Autodesk Inventor part; units mm, degrees
ref_plane "YZ Plane" through (0, 0, 0) normal (1, 0, 0) x (0, 1, 0)
ref_plane "XZ Plane" through (0, 0, 0) normal (0, 1, 0) x (-1, 0, 0)
ref_plane "XY Plane" through (0, 0, 0) normal (0, 0, 1) x (1, 0, 0)
sketch "Sketch1" plane through (0, 0, 0) normal (0, 0, 1) x (1, 0, 0)
  circle A0 centre (0, 0) radius 1.5
  circle A1 centre (-42, 0) radius 1.5
  circle A2 centre (0, -36) radius 1.5
  arc A3 (-42, 7.5) -> (-42, -7.5) centre (-42, 0) ccw
  line L0 (-42, 1.5) -> (-42, -1.5)
  arc A4 (-6, -36) -> (6, -36) centre (0, -36) ccw
  line L1 (-42, 7.5) -> (6, 7.5)
  line L2 (6, 7.5) -> (6, -36)
  line L3 (-6, -36) -> (-6, -17.5)
  line L4 (-42, -7.5) -> (-31, -7.5)
  line L5 (-31, -7.5) -> (-6, -17.5)
  dimension "d0" = 3
  dimension "d1" = 3
  dimension "d2" = 3
  dimension "d3" = 15
  dimension "d5" = 15
  dimension "d6" = 12
  dimension "d7" = 48
extrude "Extrusion1" add sketch "Sketch1" along normal blind 4
sketch "Sketch2" plane through (0, 0, 0) normal (0, 0, -1) x (-1, 0, 0)
  line L0 (6, 7.5) -> (-22, 7.5)
  line L1 (-22, -7.5) -> (6, -7.5)
  line L2 (6, -7.5) -> (6, 7.5)
  line L3 (-22, 7.5) -> (-22, -7.5)
  circle A0 centre (0, 0) radius 1.5
  dimension "d27" = 28
  dimension "d28" = 15
  dimension "d29" = 28
  dimension "d30" = 6
  dimension "d31" = 7.5
  dimension "d32" = 3
extrude "Extrusion4" add sketch "Sketch2" along normal blind 4
sketch "Sketch5" plane through (0, 0, -4) normal (0, 0, -1) x (-1, 0, 0)
  line L0 (-6, 7.5) -> (-22, 7.5)
  line L1 (-22, 7.5) -> (-10, 7.5)
  line L2 (-10, 7.5) -> (-10, -7.5)
  line L3 (-10, -7.5) -> (-22, -7.5)
  line L4 (-22, -7.5) -> (-22, 7.5)
  point P0 (0, 0)
  dimension "d35" = 12
  dimension "d36" = 15
extrude "Extrusion5" add sketch "Sketch5" along normal blind 16
shell "Shell2" thickness 4 removed faces 1 at (18, 2.5, -20)
sketch "Sketch6" plane through (0, 0, 0) normal (0, 0, -1) x (-1, 0, 0)
  circle A0 centre (12.5, 0) radius 1.5
  line L0 (6, 7.5) -> (-10, 7.5)
  point P0 (0, 0)
  dimension "d40" = 3
  dimension "d41" = 12.5
  dimension "d42" = 7.5
sketch "Sketch7" plane through (0, 0, 0) normal (0, 0, -1) x (-1, 0, 0)
  point P0 (0, 0)
extrude "Extrusion6" cut sketch "Sketch6" against normal through all
sketch "Sketch8" plane through (0, 0, 0) normal (0, 0, -1) x (-1, 0, 0)
  circle A0 centre (25.5, 0) radius 1.5
  circle A1 centre (12.5, 0) radius 1.5
  line L0 (6, 7.5) -> (-10, 7.5)
  point P0 (0, 0)
  dimension "d45" = 3
  dimension "d46" = 13
  dimension "d47" = 7.5
extrude "Extrusion7" cut sketch "Sketch8" against normal through all contours A0
sketch "Sketch9" plane through (0, 0, 0) normal (0, 0, -1) x (-1, 0, 0)
  point P0 (0, 0)
sketch "Sketch10" plane through (0, 0, 0) normal (0, 0, -1) x (-1, 0, 0)
  circle A0 centre (0, -16) radius 1.5
  line L0 (6, -36) -> (6, -17.5)
  circle A1 centre (0, -36) radius 1.5
  point P0 (0, 0)
  dimension "d50" = 3
  dimension "d51" = 6
  dimension "d52" = 20
extrude "Extrusion8" cut sketch "Sketch10" against normal through all contours A0
properties part number "Mounting Bracket 2of4 - Copy2"
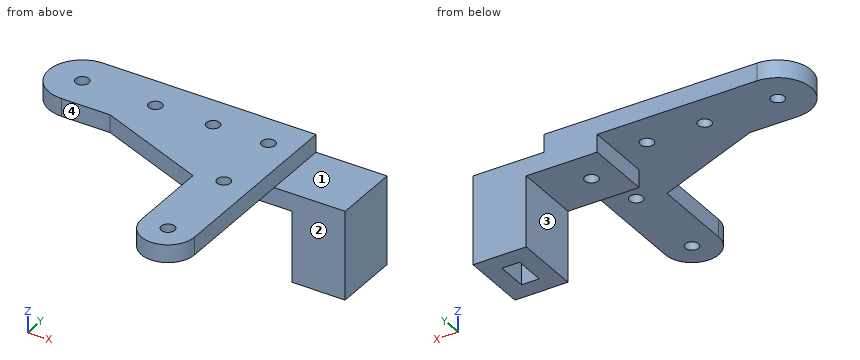
Design review of the part built by this model. Coordinates are the model's own, in mm. Face numbers are marked on the shaded views. A direction names the side the tool comes from. Coordinates: 2 decimals unless noted, no trailing zeros. Loops run counter-clockwise (first coordinate to the right, second up) from the corner with the lowest first, then second, coordinate; pieces in that order, holes last. Notation, with made-up numbers: (-7.75, 11.5) -> (5.25, 11.5) arc R38 ccw to (5.25, 49.5) -> close; hole circle Ø8 at (-31, 39.5). An arc over 180 degrees is marked (long way). Answer as a JSON object with one key per item and string values.
Q1. Clearance check with flat-ended pins moving along their axes: pin 1 Ø10 at (x, z) = (15, -6.5) entering from -Y; pin 2 Ø2 at (y, z) = (0.5, -2.5) entering from -X; pin 3 Ø2 at (y, z) = (1, -14) entering from -X; pin 4 Ø1.8 at (x, y) = (0, 0) entering from -Z. State where each tip first meets the part, or that it passes through.
Answer block:
{"pin 1": "stops at y = -7.5", "pin 2": "stops at x = -6", "pin 3": "stops at x = 10", "pin 4": "passes through"}
Q2. To check wall thickness, follow L1, parallel to Y at x = 0, z = 3; L2, parallel to Y at x = 13, z = -9; L3, parallel to Z at x = -37.5, y = 0.5. State the ranges of each line that lie inside material, in increasing order.
Answer block:
{"L1": "y = -42 to -37.5, -34.5 to -17.5, -14.5 to -1.5, 1.5 to 7.5", "L2": "y = -7.5 to 7.5", "L3": "z = 0 to 4"}
Q3. Take a section at A-A on x = -12.5. Give the boundary of the cut face in (y, z).
Answer block:
{"outline": "(-14.9, 0) -> (-1.5, 0) -> (-1.5, 4) -> (-14.9, 4) -> close; (1.5, 0) -> (7.5, 0) -> (7.5, 4) -> (1.5, 4) -> close"}
Q4. Take a section at B-B on x = 0. Give the boundary of the cut face in (y, z), plus the area to 3 significant figures.
Answer block:
{"outline": "(-42, 0) -> (-37.5, 0) -> (-37.5, 4) -> (-42, 4) -> close; (-34.5, 0) -> (-17.5, 0) -> (-17.5, 4) -> (-34.5, 4) -> close; (-14.5, 0) -> (-7.5, 0) -> (-7.5, -4) -> (-1.5, -4) -> (-1.5, 4) -> (-14.5, 4) -> close; (1.5, -4) -> (7.5, -4) -> (7.5, 4) -> (1.5, 4) -> close", "area": "210 mm^2"}
Q5. Take a section at D-D on z = -17.5. Give the boundary of the cut face in (x, y), plus the area to 3 significant figures.
Answer block:
{"outline": "(10, -7.5) -> (22, -7.5) -> (22, 7.5) -> (10, 7.5) -> close; hole (14, -3.5) -> (18, -3.5) -> (18, 3.5) -> (14, 3.5) -> close", "area": "152 mm^2"}
Q6. Take a section at C-C on y = -16. Give the boundary of the cut face in (x, z).
Answer block:
{"outline": "(-9.75, 0) -> (-1.5, 0) -> (-1.5, 4) -> (-9.75, 4) -> close; (1.5, 0) -> (6, 0) -> (6, 4) -> (1.5, 4) -> close"}
Q7. Tool access review of the marked faces 1, 2, 3 and 4: name each direction out of +Z, -Z, +X, -X, +Y, -Y from which nothing blocks a thin tool from reaching the whole face with its end or side.
Answer block:
{"face 1": "+Z, +X, +Y, -Y", "face 2": "-Z, +X, -X, -Y", "face 3": "-Z, -X, +Y, -Y", "face 4": "+Z, -Z, -X, -Y"}
